Geometry check sheet. Reference: drawing and pictorial views, mm from the part's lowest x, y, z. A direction names the side the tool comes from. Give positions to 0.01 mm unless a question says otherwise; leave off trailing zeros. Write each loop counter-clockwise with the first axis right and the second up, starting at its lowest first coordinate (ties: lowest second). Pieces come first, ordered by that corner, then holes. Notation, with made-up numbers: M 49,31 L 69,31 A33 ccw 69,62 Z; hole C -10.5,64.5 d4. An arc over 180 degrees is marked long. Write item = value, one per line. Start each with the question number.
1) Mould release check, pull along Z, two halves, no side actions. Record for the marked faces 5, 6 and 7: released by +Z, released by -Z, zero draft, split by the parting line, or undercut.
2) Go/stop test with flat-tipped pins: pin 1 (0.6 mm diameter, centred on y = 2, z = 1.5, fed in from +X); pin 2 (2 mm diameter, centred on y = 2, z = 1, fed in from -X); pin 3 (1.6 mm diameter, centred on y = 3.5, z = 9.5, fed in from +X). Record where each tip stops, or that it passes through.
3) Scan lines: line 1 along Z through (x, y) = (6.5, 1.75); line 2 along Z through (x, y) = (9, 3.75); line 3 along Y through (x, z) = (3.25, 1.5). Record each from-to range of solid material in increasing order. Write a range as [from, to].
4) Cross-section at D-D, the plane y = 8. Record the cut outline in (x, z).
5) Cross-section at A-A, the plane y = 6. Record the cut outline in (x, z), plus the area to 3 significant figures.
6) Cross-section at B-B, the plane z = 10.25. Record the cut outline in (x, y), plus the area to 3 significant figures.
7) Cross-section at C-C, the plane x = 3.5. Record the cut outline in (y, z).
8) Access from +Z, -Z, +X, -X, +Y, -Y to the whole of each face (thin tool, end or side, straight path). Record for the marked faces 1, 2, 3 and 4.
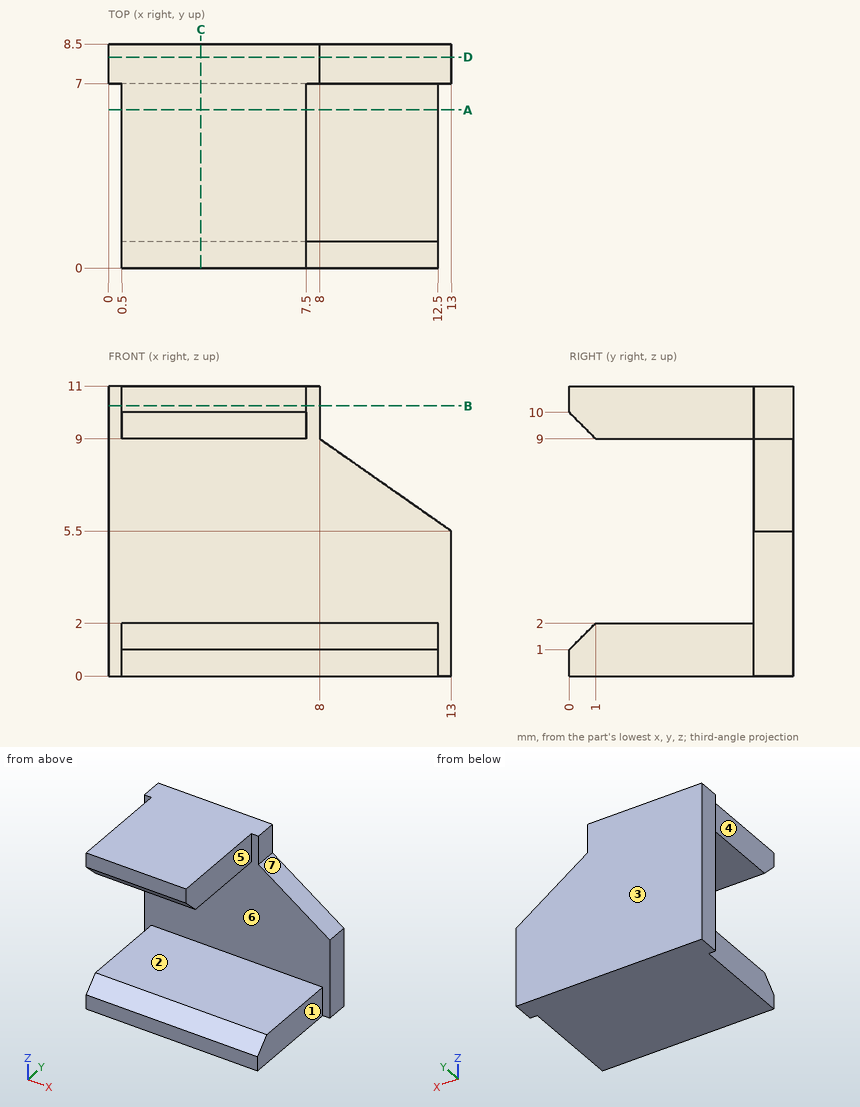
Reply:
q1.face_5 = zero draft
q1.face_6 = undercut
q1.face_7 = released by +Z
q2.pin_1 = 12.5
q2.pin_2 = 0.5
q2.pin_3 = 7.5
q3.line_1 = [0, 2], [9, 11]
q3.line_2 = [0, 2]
q3.line_3 = [0.5, 8.5]
q4.outline = M 0,0 L 13,0 L 13,5.5 L 8,9 L 8,11 L 0,11 Z
q5.outline = M 0.5,0 L 12.5,0 L 12.5,2 L 0.5,2 Z; M 0.5,9 L 7.5,9 L 7.5,11 L 0.5,11 Z
q5.area = 38.0 mm2
q6.outline = M 0,7 L 0.5,7 L 0.5,0 L 7.5,0 L 7.5,7 L 8,7 L 8,8.5 L 0,8.5 Z
q6.area = 61.0 mm2
q7.outline = M 0,0 L 8.5,0 L 8.5,11 L 0,11 L 0,10 L 1,9 L 7,9 L 7,2 L 1,2 L 0,1 Z
q8.face_1 = +Z, -Z, +X, -Y
q8.face_2 = +X, -X, -Y
q8.face_3 = +Z, -Z, +X, -X, +Y
q8.face_4 = +Z, -Z, -X, -Y
